Part print with two shaded views. Sizes in mm from the minimum x, y, z corner. Give positions to 0.01 mm unless a question says otherwise; leave off trailing zeros. Loops run counter-clockwise (first coordinate to the right, second up) from the corner with the lowest first, then second, coordinate; pieces in that order, holes last. Notation, with made-up numbers: M 31,29 L 78,29 A7 ccw 78,36 Z; hole C -36.75,30.5 d8. An arc over 180 degrees is marked long. Answer as a JSON object with one key per item and string values. Group by question number.
1. Drop flat-ended pins along their axis: pin 1 Ø1.5 at (y, z) = (17, 6.5) entering from +X; pin 2 Ø1.9 at (y, z) = (21.5, 29.5) entering from +X (3 decimals); pin 3 Ø5 at (x, z) = (12, 13.5) entering from -Y. Give the stop position or say it passes through.
2. Mould opens along Y. For the marked faces 1, 2 and 3 say: released by +Y, released by -Y, zero draft, split by the parting line, or undercut.
3. Slice it at D-D (z = 12). List the corners of the cut face in (x, y).
4. Slice it at A-A (x = 16). List the corners of the cut face in (y, z) (3 decimals).
5. Slice it at B-B (y = 59.5). List the corners of the cut face in (x, z).
6. Drill centre lines: line 1 along Y through (x, z) = (11, 12.5); line 2 along X through (y, z) = (70.5, 12); line 3 along X through (y, z) = (128.5, 15). Where is each one in solid material? Low to high. Write a range as [from, to].
7. Slice it at C-C (z = 32). List the corners of the cut face in (x, y) (3 decimals).
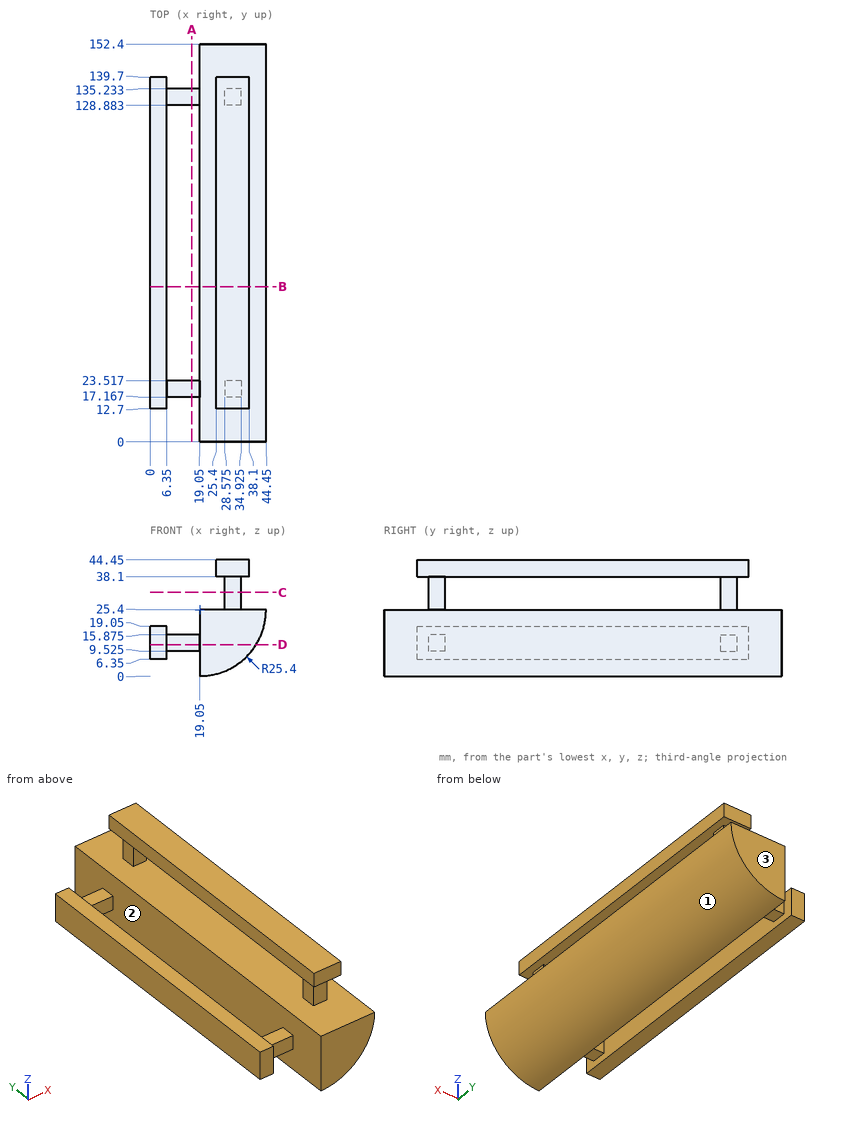
Established:
{
 "1": {"pin 1": "stops at x = 36.82", "pin 2": "stops at x = 34.925", "pin 3": "stops at y = 17.17"},
 "2": {"face 1": "zero draft", "face 2": "undercut", "face 3": "released by +Y"},
 "3": {"outline": "M 0,12.7 L 6.35,12.7 L 6.35,17.17 L 19.05,17.17 L 19.05,0 L 40.63,0 L 40.63,152.4 L 19.05,152.4 L 19.05,135.23 L 6.35,135.23 L 6.35,139.7 L 0,139.7 Z; hole M 6.35,23.52 L 19.05,23.52 L 19.05,128.88 L 6.35,128.88 Z"},
 "4": {"outline": "M 17.167,9.525 L 23.517,9.525 L 23.517,15.875 L 17.167,15.875 Z; M 128.883,9.525 L 135.233,9.525 L 135.233,15.875 L 128.883,15.875 Z"},
 "5": {"outline": "M 0,6.35 L 6.35,6.35 L 6.35,19.05 L 0,19.05 Z; M 19.05,0 A25.4 ccw 44.45,25.4 L 19.05,25.4 Z; M 25.4,38.1 L 38.1,38.1 L 38.1,44.45 L 25.4,44.45 Z"},
 "6": {"line 1": "y = [17.17, 23.52], [128.88, 135.23]", "line 2": "x = [0, 6.35], [19.05, 40.63]", "line 3": "x = [0, 6.35], [19.05, 42.22]"},
 "7": {"outline": "M 28.575,17.167 L 34.925,17.167 L 34.925,23.517 L 28.575,23.517 Z; M 28.575,128.883 L 34.925,128.883 L 34.925,135.233 L 28.575,135.233 Z"}
}
